```python
from build123d import *

# Parameters (mm, degrees)
SKETCH1_R                                 = 19.05
BILLET_DEPTH                              = 3.81
SKETCH2_R                                 = 0.6477
FIRST_LOX_HOLE_DEPTH                      = 28.208842313
BRAISING_CHAMFER_SIZE                     = 0.254
LOX_HOLE_PATTERN_COUNT                    = 7
LOX_HOLE_PATTERN_PITCH                    = 2.9972
LOX_HOLE_PATTERN_COUNT_DIR2               = 7
LOX_HOLE_PATTERN_PITCH_DIR2               = 2.9972
BRAISING_CHAMFER_OF_LOX_HOLE_PATTERN_SIZE = 0.254
SKETCH3_R                                 = 0.79375
DOWEL_HOLE_DEPTH                          = 1.5875


with BuildPart() as part:
    # Sketch1 → Billet (new body)
    with BuildSketch(Plane(origin=(0, 0, 0), x_dir=(1, 0, 0), z_dir=(0, 1, 0))):
        with Locations(Location((0, 0, 0), (0, 0, 270))):
            Circle(SKETCH1_R)
    extrude(amount=-BILLET_DEPTH)

    # Sketch2 → First Lox Hole (cut, symmetric)
    with BuildSketch(Plane(origin=(0, 0, 0), x_dir=(1, 0, 0), z_dir=(0, 1, 0))):
        with Locations(Location((8.9916, 8.9916, 0), (0, 0, 270))):
            Circle(SKETCH2_R)
    first_lox_hole = extrude(amount=FIRST_LOX_HOLE_DEPTH, both=True, mode=Mode.SUBTRACT)

    # Braising Chamfer
    braising_chamfer_edges = [part.edges().sort_by_distance(p)[0] for p in [
        (8.9916, -3.81, -9.6393),
    ]]
    chamfer(braising_chamfer_edges, length=BRAISING_CHAMFER_SIZE)

    # Lox Hole Pattern: First Lox Hole 7 × 7, 5 skipped
    with Locations(*[(-i * LOX_HOLE_PATTERN_PITCH, 0, j * LOX_HOLE_PATTERN_PITCH_DIR2) for i in range(LOX_HOLE_PATTERN_COUNT) for j in range(LOX_HOLE_PATTERN_COUNT_DIR2) if (i, j) not in ((0, 0), (2, 2), (2, 4), (3, 3), (4, 2), (4, 4))]):
        add(first_lox_hole, mode=Mode.SUBTRACT)

    # Braising Chamfer of Lox Hole Pattern
    braising_chamfer_of_lox_hole_pattern_edges = [part.edges().sort_by_distance(p)[0] for p in [
        (8.9916, -3.81, -6.6421),
        (8.9916, -3.81, -3.6449),
        (8.9916, -3.81, -0.6477),
        (8.9916, -3.81, 2.3495),
        (8.9916, -3.81, 5.3467),
        (8.9916, -3.81, 8.3439),
        (5.9944, -3.81, -9.6393),
        (5.9944, -3.81, -6.6421),
        (5.9944, -3.81, -3.6449),
        (5.9944, -3.81, -0.6477),
        (5.9944, -3.81, 2.3495),
        (5.9944, -3.81, 5.3467),
        (5.9944, -3.81, 8.3439),
        (2.9972, -3.81, -9.6393),
        (2.9972, -3.81, -6.6421),
        (2.9972, -3.81, -0.6477),
        (2.9972, -3.81, 5.3467),
        (2.9972, -3.81, 8.3439),
        (0, -3.81, -9.6393),
        (0, -3.81, -6.6421),
        (0, -3.81, -3.6449),
        (0, -3.81, 2.3495),
        (0, -3.81, 5.3467),
        (0, -3.81, 8.3439),
        (-2.9972, -3.81, -9.6393),
        (-2.9972, -3.81, -6.6421),
        (-2.9972, -3.81, -0.6477),
        (-2.9972, -3.81, 5.3467),
        (-2.9972, -3.81, 8.3439),
        (-5.9944, -3.81, -9.6393),
        (-5.9944, -3.81, -6.6421),
        (-5.9944, -3.81, -3.6449),
        (-5.9944, -3.81, -0.6477),
        (-5.9944, -3.81, 2.3495),
        (-5.9944, -3.81, 5.3467),
        (-5.9944, -3.81, 8.3439),
        (-8.9916, -3.81, -9.6393),
        (-8.9916, -3.81, -6.6421),
        (-8.9916, -3.81, -3.6449),
        (-8.9916, -3.81, -0.6477),
        (-8.9916, -3.81, 2.3495),
        (-8.9916, -3.81, 5.3467),
        (-8.9916, -3.81, 8.3439),
    ]]
    chamfer(braising_chamfer_of_lox_hole_pattern_edges, length=BRAISING_CHAMFER_OF_LOX_HOLE_PATTERN_SIZE)

    # Sketch3 → Dowel Hole (cut)
    with BuildSketch(Plane(origin=(0, -3.81, 0), x_dir=(-1, 0, 0), z_dir=(0, 1, 0))):
        with Locations(Location((0, 15.24, 0), (0, 0, 90))):
            Circle(SKETCH3_R)
        with Locations(Location((0, -15.24, 0), (0, 0, 270))):
            Circle(SKETCH3_R)
    extrude(amount=DOWEL_HOLE_DEPTH, mode=Mode.SUBTRACT)


solid = part.part
```
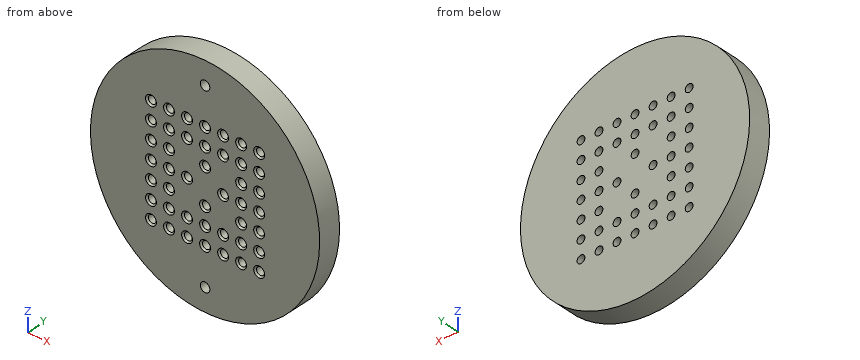
The listing builds one solid part. Answer for the finished solid, in the listing's coordinates (mm). Give positions to 0.01 mm unless a question says otherwise; leave off trailing zeros. Order: outer loops, then holes, each group sorted by start corner. A loop starts at its lowest first (then second) coordinate and runs counter-clockwise, first axis right, second up. Notation, with made-up numbers: (-9, 1.5) - (4, 1.5) arc R35 cw to (4, 38.5) - close; hole circle Ø5 at (-26, 50.5). An arc over 180 degrees is marked (long way). Use one line per item in the form item = value. Start each with the question number.
(1) A cutting plane is placed at B-B, the plane z = -15.24. Write down the section's boundary in (x, y), then the cut area to 3 significant figures.
(2) Consider line 1 (Z direction, x = 2.5, y = -2.6); line 2 (Z direction, x = 4, y = -0.3); line 3 (X direction, y = -1.45, z = -16). Determine where each line is inside the solid, lowest interval first. Write a range as from..to.
(3) A cutting plane is placed at A-A, the plane z = 0. State how many separate pieces and enclosed holes the cut face has, then the cut area to 3 significant figures.
(4) Flat-ended cylindrical pins translate along their axes: pin 1 Ø1.7 at (x, z) = (3, 5.99) entering from -Y; pin 2 Ø1.2 at (x, z) = (0, 5.99) entering from -Y (3 decimals); pin 3 Ø1.5 at (y, z) = (-1.5, -11.5) entering from +X; pin 4 Ø2 at (x, y) = (7.5, -0.5) entering from -Z. Find the tip coordinate at first contact, or state that the pin passes through.
Ans:
q1.outline = (-11.43, -3.81) - (-0.79, -3.81) - (-0.79, -2.22) - (0.79, -2.22) - (0.79, -3.81) - (11.43, -3.81) - (11.43, 0) - (-11.43, 0) - close
q1.area = 84.6 mm^2
q2.line_1 = -18.89..-9.41, -8.58..-6.41, -5.58..-0.42, 0.42..5.58, 6.41..8.58, 9.41..18.89
q2.line_2 = -18.63..18.63
q2.line_3 = -10.34..10.34
q3.separate_pieces = 7
q3.enclosed_holes = 0
q3.area = 115 mm^2
q4.pin_1 = -3.76
q4.pin_2 = through
q4.pin_3 = 15.73
q4.pin_4 = -17.91
